```python
from build123d import *

# Parameters (mm, degrees)
F0_W     = 165
F0_H     = 33
F1_DEPTH = 2
F0_W_2   = 169
F0_H_2   = 37
F2_DEPTH = 23
F0_W_3   = 20
F3_DEPTH = 23
F5_DEPTH = 209


with BuildPart() as f1:
    # F0 (on Top) → F1 (new body)
    with BuildSketch(Plane.XY):
        Rectangle(F0_W, F0_H)
    extrude(amount=F1_DEPTH)

    # F0 (on Top) → F2 (join)
    with BuildSketch(Plane.XY):
        Rectangle(F0_W_2, F0_H_2)
        Rectangle(F0_W, F0_H, mode=Mode.SUBTRACT)
    extrude(amount=F2_DEPTH)

    # F0 (on Top) → F3 (join)
    with BuildSketch(Plane.XY):
        with Locations((-94.5, 0)):
            Rectangle(F0_W_3, F0_H_2)
        with Locations((94.5, 0)):
            Rectangle(F0_W_3, F0_H_2)
    extrude(amount=F3_DEPTH)

    # F4 (on face) → F5 (join)
    with BuildSketch(Plane.YZ.offset(104.5)):
        Polygon((-63.5, 0), (-18.5, 0), (-18.5, 23), (-63.5, 5), align=None)
        Polygon((18.5, 23), (18.5, 0), (63.5, 0), (63.5, 5), align=None)
    extrude(amount=-F5_DEPTH)


solid = f1.part
```
For this review, take the finished solid that the model builds, in its own axes (mm). A direction names the side the tool comes from. Coordinates: 2 decimals unless noted, no trailing zeros. Loops run counter-clockwise (first coordinate to the right, second up) from the corner with the lowest first, then second, coordinate; pieces in that order, holes last. Notation, with made-up numbers: (13.25, 87) -> (25.25, 87) arc R15 cw to (25.25, 103) -> close; hole circle Ø11 at (-23.5, 18). An arc over 180 degrees is marked (long way). Return JSON: item names as keys, results as strings. Group by question number.
(1) Mouldability with a two-part tool opening along X and no side actions: class faces 3 (the flat face through (104.5, -1, 9)), 4 (the flat face through (0, 18, 23)), 5 (the flat face through (-82.5, 0, 12)) as pulls with the +X half, pulls with the -X half, needs draft (parallel to the pull), parting line crosses it, or undercut.
(2) For pin 1 Ø6 at (x, y) = (16, -37) entering from +Z; pin 2 Ø16.5 at (x, y) = (-27.5, -2.5) entering from +Z, all flat-tipped, find the tip position at first contact; note any pin that passes through.
(3) Tool access review of faces 1 (the flat face through (-1, 16.5, 12)), 2 (the flat face through (1, -63.5, 3)): name each direction out of +Z, -Z, +X, -X, +Y, -Y from which nothing blocks a thin tool from reaching the whole face with its end or side.
(4) Consider section D-D, the plane y = 43.5. Give the boundary of the cut face in (x, z), plus the area to 3 significant figures.
(5) Consider section A-A, the plane z = 15. Give the boundary of the cut face in (x, y), plus the area to 3 significant figures.
(6) Consider section B-B, the plane y = 14.5. Give the boundary of the cut face in (x, z).
(7) To check wall thickness, follow L1, parallel to X at y = 2, z = 21; L2, parallel to Z at x = -28.5, y = -1.5; L3, parallel to Z at x = -31, y = -20. State the ranges of each line that lie inside material, in increasing order.
(8) Consider section C-C, the plane x = -74. Give the boundary of the cut face in (y, z).
Results below:
{
 "1": {"face 3": "pulls with the +X half", "face 4": "needs draft", "face 5": "undercut"},
 "2": {"pin 1": "stops at z = 16.8", "pin 2": "stops at z = 2"},
 "3": {"face 1": "+Z", "face 2": "+Z, -Z, +X, -X, -Y"},
 "4": {"outline": "(-104.5, 0) -> (104.5, 0) -> (104.5, 13) -> (-104.5, 13) -> close", "area": "2,720 mm2"},
 "5": {"outline": "(-104.5, -38.5) -> (104.5, -38.5) -> (104.5, 38.5) -> (-104.5, 38.5) -> close; hole (-82.5, -16.5) -> (82.5, -16.5) -> (82.5, 16.5) -> (-82.5, 16.5) -> close", "area": "10,600 mm2"},
 "6": {"outline": "(-104.5, 0) -> (104.5, 0) -> (104.5, 23) -> (82.5, 23) -> (82.5, 2) -> (-82.5, 2) -> (-82.5, 23) -> (-104.5, 23) -> close"},
 "7": {"L1": "x = -104.5 to -82.5, 82.5 to 104.5", "L2": "z = 0 to 2", "L3": "z = 0 to 22.4"},
 "8": {"outline": "(-63.5, 0) -> (63.5, 0) -> (63.5, 5) -> (18.5, 23) -> (16.5, 23) -> (16.5, 2) -> (-16.5, 2) -> (-16.5, 23) -> (-18.5, 23) -> (-63.5, 5) -> close"}
}
